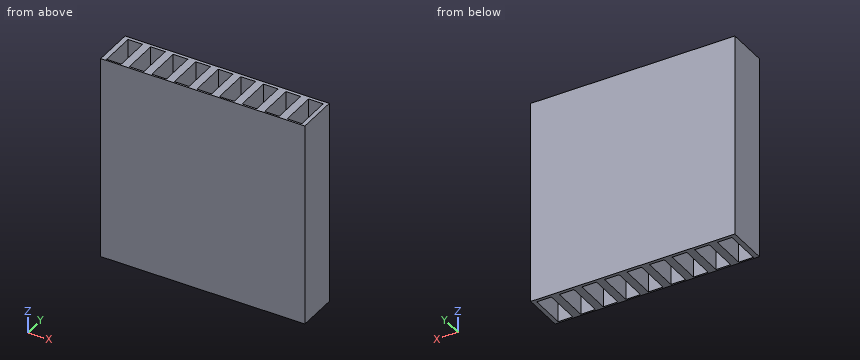
Autodesk Inventor part; units mm, degrees
ref_plane "YZ Plane" through (0, 0, 0) normal (1, 0, 0) x (0, 1, 0)
ref_plane "XZ Plane" through (0, 0, 0) normal (0, 1, 0) x (-1, 0, 0)
ref_plane "XY Plane" through (0, 0, 0) normal (0, 0, 1) x (1, 0, 0)
sketch "Sketch1" plane through (0, 0, 0) normal (0, 1, 0) x (-1, 0, 0)
  line L0 (0, 0) -> (200, 0)
  line L1 (200, 0) -> (200, 200)
  line L2 (200, 200) -> (0, 200)
  line L3 (0, 200) -> (0, 0)
  dimension "d0" = 200
  dimension "d1" = 200
extrude "Extrusion1" add sketch "Sketch1" along normal blind 40
sketch "Sketch2" plane through (0, 0, 0) normal (0, 0, -1) x (-1, 0, 0)
  line L0 (4.0349, 36.8144) -> (18.3828, 36.8144)
  line L1 (18.3828, 36.8144) -> (18.3828, 1.6542)
  line L2 (18.3828, 1.6542) -> (4.0349, 1.6542)
  line L3 (4.0349, 1.6542) -> (4.0349, 36.8144)
  point P0 (0, 0)
extrude "Extrusion2" cut sketch "Sketch2" against normal blind 310
pattern_linear "Rectangular Pattern1" count 9 spacing 22.098 along (-1, 0, 0) of "Extrusion2"
properties part number "refractory_quarry_tile"
The model under review builds one solid part; all positions refer to its coordinate system, in mm. Round coordinates to 2 decimals unless told otherwise and drop trailing zeros. Loops run counter-clockwise (first coordinate to the right, second up) from the corner with the lowest first, then second, coordinate; pieces in that order, holes last. Notation, with made-up numbers: (-1.5, 31) -> (26.5, 31) arc R21 cw to (26.5, 52) -> close; hole circle Ø11 at (-14.75, -9). An arc over 180 degrees is marked (long way). Answer in a Markdown table with one row per item.
1) Consider section A-A, the plane x = -148.5. Write out the cut boundary in (y, z), plus the area to 3 significant figures.
Taken from the geometry:
| item | result |
|---|---|
| outline | (0, 0) -> (1.65, 0) -> (1.65, 200) -> (0, 200) -> close; (36.81, 0) -> (40, 0) -> (40, 200) -> (36.81, 200) -> close |
| area | 968 mm² |
2) Wall thickness on line 1 along Y through (x, z) = (-39, 25.5): over which ranges is the line inside the solid? List them lowest first.
Taken from the geometry:
| item | result |
|---|---|
| line 1 | y = 0 to 1.65, 36.81 to 40 |
3) Consider section B-B, the plane y = 12. Count the separate pieces of the cut face and the enclosed holes in it, plus the area to 3 significant figures.
Taken from the geometry:
| item | result |
|---|---|
| separate pieces | 10 |
| enclosed holes | 0 |
| area | 14,200 mm² |
